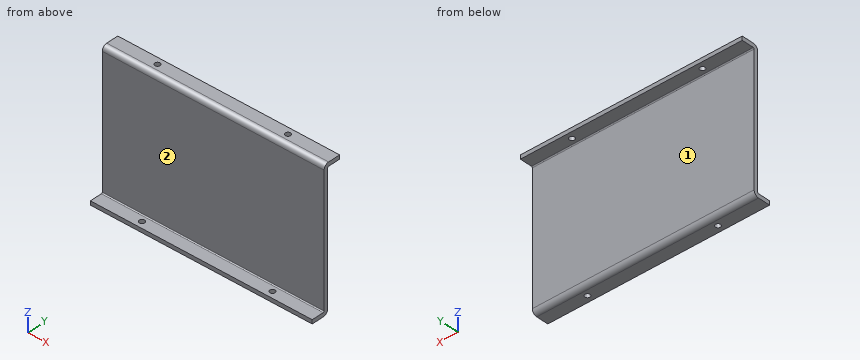
from build123d import *

# Parameters (mm, degrees)
SKETCH_1_W                       = 170
SKETCH_1_H                       = 100
SM_BASE_FLANGE_1_DEPTH           = 3
SM_EDGE_FLANGE_3_STRIP_W         = 13.4732
SM_EDGE_FLANGE_3_STRIP_H         = 3
SM_EDGE_FLANGE_3_STRIP_CUT_DEPTH = 170
SM_EDGE_FLANGE_3_DEPTH           = 170
SM_EDGE_FLANGE_4_STRIP_W         = 13.4732
SM_EDGE_FLANGE_4_STRIP_H         = 3
SM_EDGE_FLANGE_4_STRIP_CUT_DEPTH = 170
SM_EDGE_FLANGE_4_DEPTH           = 170
CUT_EXTRUDE_2_REACH              = 138.492
SKETCH_19_R                      = 2
CUT_EXTRUDE_3_REACH              = 138.492
SKETCH_20_R                      = 2


# Sheet-metal steps are written as plain solids
with BuildPart() as part:
    # Sketch 1 → 基体-法兰1 (new body)
    with BuildSketch(Plane(origin=(0, 0, 0), x_dir=(1, 0, 0), z_dir=(0, 1, 0))):
        Rectangle(SKETCH_1_W, SKETCH_1_H)
    extrude(amount=-SM_BASE_FLANGE_1_DEPTH)

    # 边线-法兰3 strip (across the edge) → 边线-法兰3 strip cut (cut)
    with BuildSketch(Plane(origin=(-85, 0, 50), x_dir=(0, 0, -1), z_dir=(1, 0, 0))):
        with Locations((-6, -1.5)):
            Rectangle(SM_EDGE_FLANGE_3_STRIP_W, SM_EDGE_FLANGE_3_STRIP_H)
    extrude(amount=SM_EDGE_FLANGE_3_STRIP_CUT_DEPTH, mode=Mode.SUBTRACT)

    # 边线-法兰3 section (across the edge) → 边线-法兰3 (add)
    with BuildSketch(Plane(origin=(-85, 0, 50), x_dir=(0, 0, -1), z_dir=(1, 0, 0))):
        with BuildLine():
            Line((-3, 0.7366), (-3, 10))
            Line((-3, 10), (0, 10))
            Line((0, 10), (0, 0.7366))
            ThreePointArc((0, 0.7366), (0.215745145, 0.215745145), (0.7366, 0))
            Line((0.7366, 0), (0.7366, -3))
            ThreePointArc((0.7366, -3), (-1.905575199, -1.905575199), (-3, 0.7366))
        make_face()
    extrude(amount=SM_EDGE_FLANGE_3_DEPTH)

    # 边线-法兰4 strip (across the edge) → 边线-法兰4 strip cut (cut)
    with BuildSketch(Plane(origin=(-85, -3, -50), x_dir=(0, 0, 1), z_dir=(1, 0, 0))):
        with Locations((-6, -1.5)):
            Rectangle(SM_EDGE_FLANGE_4_STRIP_W, SM_EDGE_FLANGE_4_STRIP_H)
    extrude(amount=SM_EDGE_FLANGE_4_STRIP_CUT_DEPTH, mode=Mode.SUBTRACT)

    # 边线-法兰4 section (across the edge) → 边线-法兰4 (add)
    with BuildSketch(Plane(origin=(-85, -3, -50), x_dir=(0, 0, 1), z_dir=(1, 0, 0))):
        with BuildLine():
            Line((-3, 0.7366), (-3, 10))
            Line((-3, 10), (0, 10))
            Line((0, 10), (0, 0.7366))
            ThreePointArc((0, 0.7366), (0.215745145, 0.215745145), (0.7366, 0))
            Line((0.7366, 0), (0.7366, -3))
            ThreePointArc((0.7366, -3), (-1.905575199, -1.905575199), (-3, 0.7366))
        make_face()
    extrude(amount=SM_EDGE_FLANGE_4_DEPTH)

    # 草图19 → 切除-拉伸2 (cut, up to next)
    with BuildSketch(Plane.XY.offset(53), mode=Mode.PRIVATE) as cut_extrude_2_sk1:
        with Locations((-50, 5)):
            Circle(SKETCH_19_R)
    cut_extrude_2_tool1 = extrude(cut_extrude_2_sk1.sketch, amount=-CUT_EXTRUDE_2_REACH, mode=Mode.PRIVATE) & part.part
    # 草图19 → 切除-拉伸2 (cut, up to next)
    with BuildSketch(Plane.XY.offset(53), mode=Mode.PRIVATE) as cut_extrude_2_sk2:
        with Locations((50, 5)):
            Circle(SKETCH_19_R)
    cut_extrude_2_tool2 = extrude(cut_extrude_2_sk2.sketch, amount=-CUT_EXTRUDE_2_REACH, mode=Mode.PRIVATE) & part.part
    add(cut_extrude_2_tool1.solids().sort_by_distance((-50, 5, 53))[0], mode=Mode.SUBTRACT)
    add(cut_extrude_2_tool2.solids().sort_by_distance((50, 5, 53))[0], mode=Mode.SUBTRACT)

    # 草图20 → 切除-拉伸3 (cut, up to next)
    with BuildSketch(Plane(origin=(0, 0, -53), x_dir=(-1, 0, 0), z_dir=(0, 0, -1)), mode=Mode.PRIVATE) as cut_extrude_3_sk1:
        with Locations(Location((-50, -8, 0), (0, 0, 90))):
            Circle(SKETCH_20_R)
    cut_extrude_3_tool1 = extrude(cut_extrude_3_sk1.sketch, amount=-CUT_EXTRUDE_3_REACH, mode=Mode.PRIVATE) & part.part
    # 草图20 → 切除-拉伸3 (cut, up to next)
    with BuildSketch(Plane(origin=(0, 0, -53), x_dir=(-1, 0, 0), z_dir=(0, 0, -1)), mode=Mode.PRIVATE) as cut_extrude_3_sk2:
        with Locations(Location((50, -8, 0), (0, 0, 90))):
            Circle(SKETCH_20_R)
    cut_extrude_3_tool2 = extrude(cut_extrude_3_sk2.sketch, amount=-CUT_EXTRUDE_3_REACH, mode=Mode.PRIVATE) & part.part
    add(cut_extrude_3_tool1.solids().sort_by_distance((50, -8, -53))[0], mode=Mode.SUBTRACT)
    add(cut_extrude_3_tool2.solids().sort_by_distance((-50, -8, -53))[0], mode=Mode.SUBTRACT)


solid = part.part
Work out the finished part from the listing and answer in its coordinate system (mm). Face numbers are marked on the shaded views. A direction names the side the tool comes from. Coordinates: 2 decimals unless noted, no trailing zeros. Loops run counter-clockwise (first coordinate to the right, second up) from the corner with the lowest first, then second, coordinate; pieces in that order, holes last. Notation, with made-up numbers: M 73.25,-36 L 113.25,-36 A36 cw 113.25,1 Z; hole C 85.5,21 d11. An arc over 180 degrees is marked long. Answer in a Markdown table with one row per item. Add a question column.
1. Find section C-C, the plane z = 28. Write down the section's boundary in (x, y).
2. A tool of negligible diameter and unlimited length cuts with its end or side. For the marked faces 1 and 2, from which of +Z, -Z, +X, -X, +Y, -Y can it reach the whole face along a straight path? Write none if from no direction.
3. Find section B-B, the plane y = 5. Write down the section's boundary in (x, z).
4. Flat-ended cylindrical pins translate along their axes: P1, Ø8, axis at x = 21, z = 5, coming from the -Y side; P2, Ø1.5, axis at x = -41.5, y = -7, coming from the +Z side; P3, Ø12, axis at x = 25.5, z = 39.5, coming from the +Y side. Find the tip coordinate at first contact, or state that the pin passes through.
5. Consider L1, parallel to X at y = -8, z = -51.25; L2, parallel to Y at x = 30, z = -8.5; L3, parallel to Z at x = -73, y = 8.25. Determine where each line is inside the solid, lowest interval first.
6. Find section A-A, the plane x = 50. Write down the section's boundary in (y, z).
Reported:
| question | item | result |
|---|---|---|
| 1 | outline | M -85,-3 L 85,-3 L 85,0 L -85,0 Z |
| 2 | face 1 | -Z, +X, -X, +Y |
| 2 | face 2 | +Z, +X, -X, -Y |
| 3 | outline | M -85,50 L -52,50 L -52,53 L -85,53 Z; M -48,50 L 48,50 L 48,53 L -48,53 Z; M 52,50 L 85,50 L 85,53 L 52,53 Z |
| 4 | P1 | stops at y = -3 |
| 4 | P2 | stops at z = -50 |
| 4 | P3 | stops at y = 0 |
| 5 | L1 | x = -85 to -52, -48 to 48, 52 to 85 |
| 5 | L2 | y = -3 to 0 |
| 5 | L3 | z = 50 to 53 |
| 6 | outline | M -13,-53 L -10,-53 L -10,-50 L -13,-50 Z; M -6,-53 L -3.74,-53 A3.74 ccw 0,-49.26 L 0,49.26 A0.74 cw 0.74,50 L 3,50 L 3,53 L 0.74,53 A3.74 ccw -3,49.26 L -3,-49.26 A0.74 cw -3.74,-50 L -6,-50 Z; M 7,50 L 10,50 L 10,53 L 7,53 Z |
